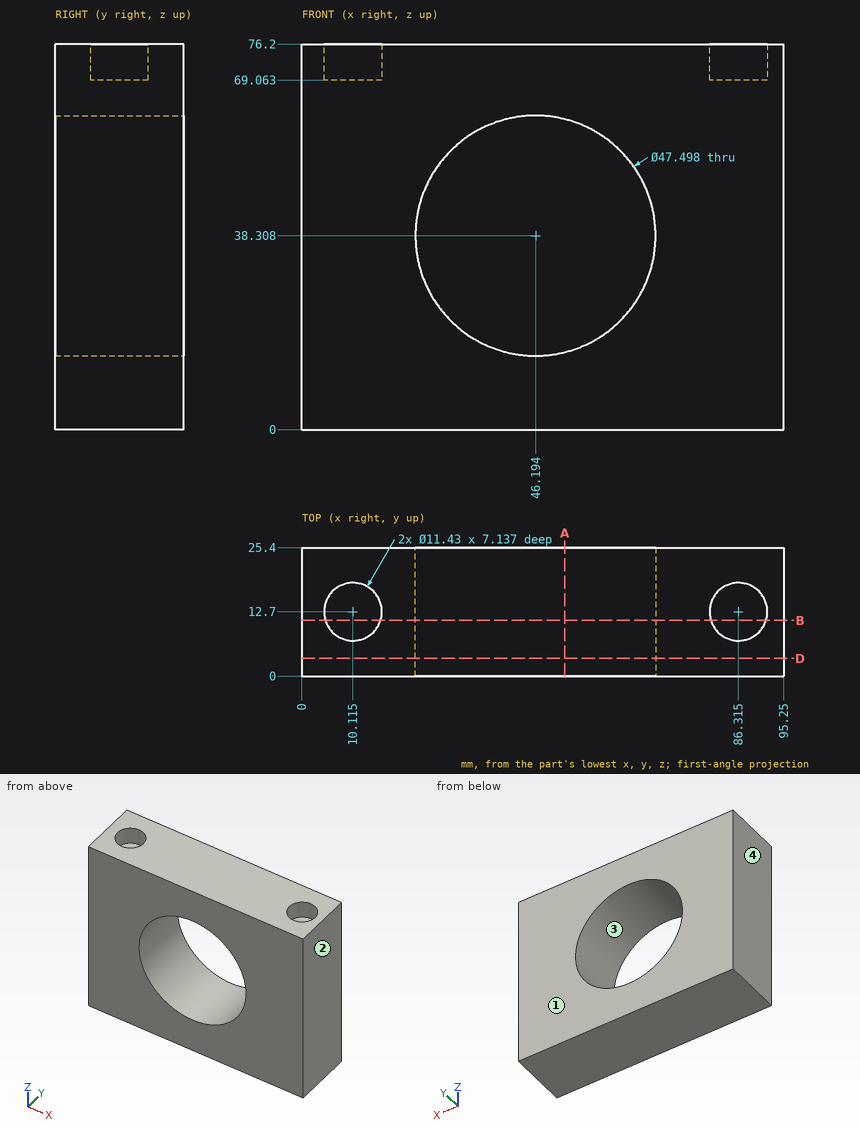
Source: three-view drawing plus pictorial views. Frame: mm from the lowest corner of the part. Give positions to 0.01 mm unless a question says otherwise; leave off trailing zeros. Write each loop counter-clockwise with the first axis right and the second up, starting at its lowest first coordinate (ties: lowest second). Pieces come first, ordered by that corner, then holes. Notation, with made-up numbers: (-37, 30) -> (-18, 30) arc R20 cw to (-18, 58) -> close; hole circle Ø7 at (52, -27.75). An arc over 180 degrees is marked (long way). Write item = value, one per line.
Q1. Cut plane D-D on y = 3.5. Return loops of the section in (x, z), then the cut area to 3 significant figures.
Here are the results:
outline = (0, 0) -> (95.25, 0) -> (95.25, 76.2) -> (0, 76.2) -> close; hole circle Ø47.5 at (46.19, 38.31)
area = 5,490 mm²
Q2. First-contact query: pin 1 (3.5 mm diameter, centred on x = 83.5, y = 11.5, fed in from +Z). Flat tip, straight axial feed; report the tip coordinate or a pass-through.
Here are the results:
pin_1 = 69.06
Q3. Mould query, pull axis X, two halves, no side actions, for the marked faces 1, 2, 3 and 4. Classes: +X half, -X half, draft (parallel to the pull), parting line (faces both ways), or undercut.
Here are the results:
face_1 = draft
face_2 = +X half
face_3 = undercut
face_4 = -X half
Q4. Line query: line 1 (X direction, y = 10.25, z = 72); line 2 (Z direction, x = 37, y = 17.5) (1 decimal); line 3 (Z direction, x = 58, y = 1.25) (1 decimal). Output: solid intervals per line, ascending. Write a range as from..to.
Here are the results:
line_1 = 0..4.95, 15.28..81.15, 91.48..95.25
line_2 = 0..16.4, 60.2..76.2
line_3 = 0..17.7, 58.9..76.2
Q5. Cut plane B-B on y = 11. Return loops of the section in (x, z), then the cut area to 3 significant figures.
Here are the results:
outline = (0, 0) -> (95.25, 0) -> (95.25, 76.2) -> (91.77, 76.2) -> (91.77, 69.06) -> (80.86, 69.06) -> (80.86, 76.2) -> (15.57, 76.2) -> (15.57, 69.06) -> (4.66, 69.06) -> (4.66, 76.2) -> (0, 76.2) -> close; hole circle Ø47.5 at (46.19, 38.31)
area = 5,330 mm²
Q6. Cut plane A-A on x = 52. Return loops of the section in (y, z), then the cut area to 3 significant figures.
Here are the results:
outline = (0, 0) -> (25.4, 0) -> (25.4, 15.28) -> (0, 15.28) -> close; (0, 61.34) -> (25.4, 61.34) -> (25.4, 76.2) -> (0, 76.2) -> close
area = 766 mm²
